from build123d import *

# Parameters (mm, degrees)
F1_DEPTH = 5.08


with BuildPart() as f1:
    # F0 (on Top) → F1 (new body)
    with BuildSketch(Plane.XY):
        Polygon((0.478612, 7.462469), (0, 6.012231), (-1.523086, 5.815863), (-2.353894, 7.097243), (-3.241167, 6.738036), (-2.946527, 5.239563), (-3.591382, 4.819802), (-4.842358, 5.695772), (-5.529986, 5.02986), (-4.694555, 3.751453), (-5.134762, 3.12039), (-6.623025, 3.462909), (-7.010476, 2.5876), (-5.756377, 1.716126), (-5.927598, 0.965987), (-7.435621, 0.724967), (-7.466305, -0.23175), (-5.976798, -0.568909), (-5.854014, -1.328471), (-7.161378, -2.117801), (-6.830797, -3.016123), (-5.323637, -2.769667), (-4.924781, -3.427628), (-5.840374, -4.649876), (-5.19684, -5.358511), (-3.892321, -4.564482), (-3.275686, -5.024679), (-3.665728, -6.501206), (-2.803296, -6.916522), (-1.892071, -5.690997), (-1.147826, -5.886171), (-0.955243, -7.401128), (0, -7.462469), (0.384708, -5.984545), (1.147826, -5.886171), (1.89484, -7.218147), (2.803296, -6.916522), (2.605278, -5.40225), (3.275711, -5.024679), (4.467987, -5.979008), (5.19684, -5.358511), (4.445051, -4.029202), (4.924781, -3.427628), (6.388049, -3.864788), (6.830797, -3.016123), (5.635092, -2.066087), (5.854014, -1.328471), (7.374382, -1.184554), (7.466305, -0.23175), (6.001487, 0.200127), (5.927598, 0.965987), (7.282866, 1.669923), (7.010502, 2.5876), (5.490642, 2.438222), (5.134762, 3.12039), (6.12681, 4.281475), (5.529986, 5.02986), (4.177284, 4.321048), (3.591408, 4.819802), (4.075227, 6.268314), (3.241167, 6.738036), (2.25331, 5.573395), (1.523086, 5.815863), (1.427988, 7.340067), align=None)
        Polygon((-1.231849, 3.118993), (-0.760552, 2.969895), (-0.419405, 3.327578), (0, 3.065983), (0.419405, 3.327578), (0.760578, 2.969895), (1.231849, 3.118993), (1.473352, 2.687676), (1.9669, 2.714879), (2.093544, 2.23708), (2.578379, 2.140687), (2.582215, 1.646403), (3.027832, 1.432458), (2.90863, 0.952729), (3.287039, 0.634695), (3.052267, 0.199695), (3.339694, -0.202438), (3.004134, -0.565404), (3.182518, -1.026389), (2.767228, -1.294486), (2.825369, -1.785366), (2.35646, -1.941754), (2.290699, -2.431669), (1.797634, -2.466543), (1.612087, -2.924708), (1.12583, -2.835859), (0.832206, -3.233496), (0.383311, -3.026512), (0, -3.338627), (-0.383311, -3.026512), (-0.83218, -3.233496), (-1.12583, -2.835859), (-1.612087, -2.924708), (-1.797609, -2.466543), (-2.290699, -2.431669), (-2.35646, -1.941754), (-2.825369, -1.785366), (-2.767228, -1.294486), (-3.182518, -1.026389), (-3.004134, -0.565404), (-3.339694, -0.202438), (-3.052267, 0.199695), (-3.287014, 0.634695), (-2.908605, 0.952729), (-3.027807, 1.432458), (-2.582215, 1.646403), (-2.578354, 2.140687), (-2.093544, 2.23708), (-1.9669, 2.714879), (-1.473352, 2.687676), align=None, mode=Mode.SUBTRACT)
    extrude(amount=F1_DEPTH)


solid = f1.part
Could you check a few things on this model? Use its own coordinates, in mm. A direction names the side the tool comes from. Round coordinates to 2 decimals unless told otherwise and drop trailing zeros. Loops run counter-clockwise (first coordinate to the right, second up) from the corner with the lowest first, then second, coordinate; pieces in that order, holes last. Notation, with made-up numbers: (64.25, -21) - (111.25, -21) arc R30 ccw to (111.25, 12) - close; hole circle Ø10 at (42, -40). An arc over 180 degrees is marked (long way). Write item = value, one per line.
1) On a 3-axis mill with a long thin cutter (end or side, diameter ignored), from which of +Z, -Z, +X, -X, +Y, -Y can I reach the whole of each face in a straight line? I mean faces 1 (the flat face through (6.744, -0.019, 2.504)), 2 (the flat face through (2.706, -6.17, 2.504)), 3 (the flat face through (-3.241, -6.706, 2.504)), 4 (the flat face through (0.243, 6.748, 2.504)), 5 (the flat face through (-4.554, -4.967, 2.504)). Say none if no direction works.
Computed:
face_1 = +Z, -Z, +X
face_2 = +Z, -Z
face_3 = +Z, -Z, -X, -Y
face_4 = +Z, -Z, +Y
face_5 = +Z, -Z, -Y
2) I need wall thicknesses on line 1 along X through (y, z) = (-6.25, 4.25); line 2 along Y through (x, z) = (-6.5, 2.45); line 3 along Y through (x, z) = (-4.75, 3.9). Which ranges of each line are inside material? Lowest first, please. Write a range as from..to.
Computed:
line_1 = -3.6..-2.31, -1.1..0.32, 1.35..2.72
line_2 = -2.96..-1.72, -0.45..0.87, 2.23..3.43
line_3 = -5.09..3.67, 3.84..5.63
3) If we mould it in two halves opening along Y, with no side actions, what happens to faces 6 (the flat face through (-6.814, 3.031, 2.504)), 7 (the flat face through (6.606, -3.446, 2.504)), 8 (the flat face through (-5.87, 3.29, 2.5))? For each: pulls with the +Y half, pulls with the -Y half, needs draft (parallel to the pull), parting line crosses it, or undercut.
Computed:
face_6 = pulls with the +Y half
face_7 = pulls with the -Y half
face_8 = undercut
4) Imagine slicing it at A-A (x = -6.25). Please give me the cut outline in (y, z), and give its area (3 significant figures).
Computed:
outline = (-2.92, 0) - (-1.57, 0) - (-1.57, 5.08) - (-2.92, 5.08) - close; (-0.51, 0) - (0.91, 0) - (0.91, 5.08) - (-0.51, 5.08) - close; (2.06, 0) - (3.38, 0) - (3.38, 5.08) - (2.06, 5.08) - close
area = 20.8 mm2
5) I'm going to push flat-ended pins straight in: P1, Ø1, axis at x = 4, z = 4, coming from the -Y side; P2, Ø1, axis at x = -3, z = 3.5, coming from the -Y side. Where does each tip first touch, or does it pass through?
Computed:
P1 = -5.98
P2 = -6.92
